Part model, mm, in its own coordinate system. A direction names the side the tool comes from. Round coordinates to 2 decimals unless told otherwise and drop trailing zeros. Order: outer loops, then holes, each group sorted by start corner. A loop starts at its lowest first (then second) coordinate and runs counter-clockwise, first axis right, second up. Notation, with made-up numbers: (15.25, 51) -> (24.25, 51) arc R17 cw to (24.25, 72) -> close; hole circle Ø8 at (70, 40). An arc over 180 degrees is marked (long way). Return JSON: item names as keys, results as strings. Group by question number.
Autodesk Inventor part; units mm, degrees
ref_plane "YZ Plane" through (0, 0, 0) normal (1, 0, 0) x (0, 1, 0)
ref_plane "XZ Plane" through (0, 0, 0) normal (0, 1, 0) x (-1, 0, 0)
ref_plane "XY Plane" through (0, 0, 0) normal (0, 0, 1) x (1, 0, 0)
sketch "Sketch1" plane through (0, 0, 0) normal (1, 0, 0) x (0, 1, 0)
  line L0 (-7.5, 7.5) -> (7.5, 7.5)
  line L1 (7.5, 7.5) -> (7.5, -7.5)
  line L2 (7.5, -7.5) -> (-7.5, -7.5)
  line L3 (-7.5, -7.5) -> (-7.5, 7.5)
  line L4 (-7.5, 7.5) -> (7.5, -7.5) construction
  line L5 (7.5, 7.5) -> (-7.5, -7.5) construction
  line L6 (-6.5, 6.5) -> (6.5, 6.5)
  line L7 (6.5, 6.5) -> (6.5, -6.5)
  line L8 (6.5, -6.5) -> (-6.5, -6.5)
  line L9 (-6.5, -6.5) -> (-6.5, 6.5)
  line L10 (-6.5, 6.5) -> (6.5, -6.5) construction
  line L11 (6.5, 6.5) -> (-6.5, -6.5) construction
  point P0 (0, 0)
  dimension "d0" = 15
  dimension "d1" = 15
  dimension "d2" = 13
  dimension "d3" = 13
extrude "Extrusion1" add sketch "Sketch1" along normal blind 110
sketch "Sketch2" plane through (0, 7.5, 7.5) normal (0, 1, 0) x (1, 0, 0)
  line L0 (0, 7.5) -> (4, 7.5)
  circle A0 centre (4, 7.5) radius 1.5
  dimension "d6" = 4
  dimension "d7" = 3
extrude "Extrusion2" cut sketch "Sketch2" against normal through all
sketch "Sketch3" plane through (0, -7.5, -7.5) normal (0, -1, 0) x (1, 0, 0)
  line L0 (110, 1) -> (110, 14)
  line L1 (110, 7.5) -> (105, 7.5)
  circle A0 centre (105, 7.5) radius 1.5
  point P0 (0, 7.5)
  dimension "d10" = 5
  dimension "d11" = 3
extrude "Extrusion3" cut sketch "Sketch3" against normal through all
properties part number "front_arm_rect" material "Aluminum 6061"
(1) Mould opens along Z. For faces 3 (the flat face through (54, 0, 7.5)), 4 (the flat face through (54, 0, 6.5)), 5 (the flat face through (110, -7, 0)) say: pulls with the +Z half, pulls with the -Z half, needs draft (parallel to the pull), parting line crosses it, or undercut.
(2) Saw through at B-B, the plane z = 0. List the corners of the cut face in (x, y).
(3) Probe L1, parallel to Z at x = 83, y = -1.5; L2, parallel to Z at x = 105, y = 6.8. List the from-to ranges inside material, lowest first. Write a range as [from, to].
(4) Tool access for faces 1 (the flat face through (54, -6.5, 0)), 2 (the flat face through (54, -7.5, 0)): list every direction of +Z, -Z, +X, -X, +Y, -Y with a clear straight run to the whole face (end or side of a thin tool).
(5) Saw through at A-A, the plane y = -0.75. List the corners of the cut face in (x, z).
(6) Saw through at C-C, the plane x = 93.5. List the corners of the cut face in (y, z), and give its area (3 significant figures).
(7) Saw through at D-D, the plane x = 4. List the corners of the cut face in (y, z), and give its area (3 significant figures).
Results are:
{
 "1": {"face 3": "pulls with the +Z half", "face 4": "undercut", "face 5": "needs draft"},
 "2": {"outline": "(0, -7.5) -> (2.5, -7.5) -> (2.5, -6.5) -> (0, -6.5) -> close; (0, 6.5) -> (2.5, 6.5) -> (2.5, 7.5) -> (0, 7.5) -> close; (5.5, -7.5) -> (103.5, -7.5) -> (103.5, -6.5) -> (5.5, -6.5) -> close; (5.5, 6.5) -> (103.5, 6.5) -> (103.5, 7.5) -> (5.5, 7.5) -> close; (106.5, -7.5) -> (110, -7.5) -> (110, -6.5) -> (106.5, -6.5) -> close; (106.5, 6.5) -> (110, 6.5) -> (110, 7.5) -> (106.5, 7.5) -> close"},
 "3": {"L1": "z = [-7.5, -6.5], [6.5, 7.5]", "L2": "z = [-7.5, -1.5], [1.5, 7.5]"},
 "4": {"face 1": "+X, -X", "face 2": "+Z, -Z, +X, -X, -Y"},
 "5": {"outline": "(0, -7.5) -> (110, -7.5) -> (110, -6.5) -> (0, -6.5) -> close; (0, 6.5) -> (110, 6.5) -> (110, 7.5) -> (0, 7.5) -> close"},
 "6": {"outline": "(-7.5, -7.5) -> (7.5, -7.5) -> (7.5, 7.5) -> (-7.5, 7.5) -> close; hole (-6.5, -6.5) -> (6.5, -6.5) -> (6.5, 6.5) -> (-6.5, 6.5) -> close", "area": "56.0 mm^2"},
 "7": {"outline": "(-7.5, -7.5) -> (7.5, -7.5) -> (7.5, -1.5) -> (6.5, -1.5) -> (6.5, -6.5) -> (-6.5, -6.5) -> (-6.5, -1.5) -> (-7.5, -1.5) -> close; (-7.5, 1.5) -> (-6.5, 1.5) -> (-6.5, 6.5) -> (6.5, 6.5) -> (6.5, 1.5) -> (7.5, 1.5) -> (7.5, 7.5) -> (-7.5, 7.5) -> close", "area": "50.0 mm^2"}
}
